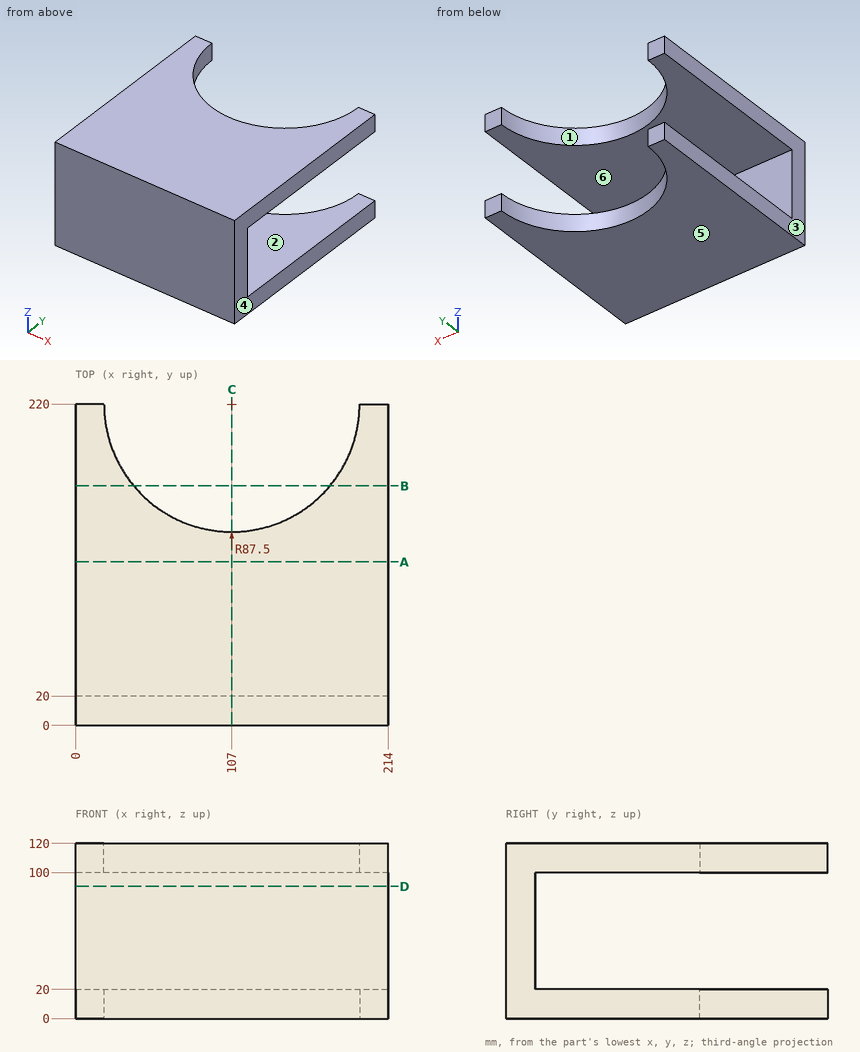
Geometry: see drawing. Coordinates: mm, zero at the bounding-box minimum. A direction names the side the tool comes from. Give positions to 0.01 mm unless a question says otherwise; leave off trailing zeros. Loops run counter-clockwise (first coordinate to the right, second up) from the corner with the lowest first, then second, coordinate; pieces in that order, holes last. Notation, with made-up numbers: (-35, -2) -> (-24, -2) arc R33 ccw to (-24, 32) -> close; hole circle Ø4 at (1, -18). An arc over 180 degrees is marked (long way). Answer as a JSON object with one key per item and string values. Group by question number.
Item 1: Reachability of the marked faces 5 and 6 from +Z, -Z, +X, -X, +Y, -Y: full face, straight path, thin tool, end or side. Return the list, or none.
Item 2: Cut plane B-B, the plane y = 164. Return the cut outline in (x, z).
Item 3: Pull-direction query (X, two-part tool) for the marked faces 1, 2, 3 and 4; classes: released by +X, released by -X, zero draft, split by the parting line, or undercut.
Item 4: Line query: probe 1 along Z at (x, y) = (132, 89); probe 2 along Y at (x, z) = (93, 82.5); probe 3 along X at (y, z) = (164, 9.5). Output: solid intervals per line, ascending.
Item 5: Cut plane C-C, the plane x = 107. Return the cut outline in (y, z).
Item 6: Cut plane D-D, the plane z = 90.5. Return the cut outline in (x, y), and give its area (3 significant figures).
Item 7: Pin query (flat end, axial travel): P1, Ø1.5, axis at y = 40.5, z = 22, coming from the +X side; P2, Ø2, axis at x = 162, z = 66, coming from the +Y side. Return the tip coordinate at first contact, or that it passes through.
Item 8: Cut plane A-A, the plane y = 112. Return the cut outline in (x, z), and give its area (3 significant figures).
Checks:
{
 "1": {"face 5": "-Z, +X, -X, +Y, -Y", "face 6": "+X, -X, +Y"},
 "2": {"outline": "(0, 0) -> (39.77, 0) -> (39.77, 20) -> (0, 20) -> close; (0, 100) -> (39.77, 100) -> (39.77, 120) -> (0, 120) -> close; (174.23, 0) -> (214, 0) -> (214, 20) -> (174.23, 20) -> close; (174.23, 100) -> (214, 100) -> (214, 120) -> (174.23, 120) -> close"},
 "3": {"face 1": "undercut", "face 2": "zero draft", "face 3": "released by -X", "face 4": "released by +X"},
 "4": {"probe 1": "z = 0 to 20, 100 to 120", "probe 2": "y = 0 to 20", "probe 3": "x = 0 to 39.77, 174.23 to 214"},
 "5": {"outline": "(0, 0) -> (132.5, 0) -> (132.5, 20) -> (20, 20) -> (20, 100) -> (132.5, 100) -> (132.5, 120) -> (0, 120) -> close"},
 "6": {"outline": "(0, 0) -> (214, 0) -> (214, 20) -> (0, 20) -> close", "area": "4,280 mm²"},
 "7": {"P1": "passes through", "P2": "stops at y = 20"},
 "8": {"outline": "(0, 0) -> (214, 0) -> (214, 20) -> (0, 20) -> close; (0, 100) -> (214, 100) -> (214, 120) -> (0, 120) -> close", "area": "8,560 mm²"}
}
